```python
from build123d import *

# Parameters (mm, degrees)
SKETCH3_R                       = 4.7625
OXIDIZER_INLET_HOLE_DEPTH       = 102.060803604
FLANGE_HOLES_D                  = 5.1054
DOWEL_HOLES_D                   = 4.7625
DOWEL_HOLES_DEPTH               = 6.35
DOWEL_HOLES_TIP                 = 1.430799349
SKETCH12_R                      = 38.1
IMPINGING_PLATE_FLAT_CUT_DEPTH  = 3.81
SKETCH14_R                      = 38.1
SKETCH15_R                      = 38.1
SKETCH16_R                      = 28.575
SKETCH17_R                      = 4.7625
SKETCH21_R                      = 28.575
CUT_EXTRUDE1_DEPTH              = 9.525
INTERNAL_FILLET_R               = 3.175
EXTENDED_8_BC_COUNT             = 8
CHAMFER_FOR_IMPINGING_EDGE_SIZE = 0.127


with BuildPart() as part:
    # Sketch2 → Main Structure (revolve)
    with BuildSketch(Plane.XY, mode=Mode.PRIVATE) as main_structure_sk:
        Polygon((0, 0), (0, 63.5), (9.525, 63.5), (9.525, 45.72), (19.05, 45.72), (31.75, 13.081), (41.355, 13.081), (41.355, 6.2484), (46.355, 6.2484), (46.355, 0), align=None)
    revolve(main_structure_sk.sketch.rotate(Axis((0, 0, 0), (1, 0, 0)), 90), axis=Axis((0, 0, 0), (1, 0, 0)))

    # Sketch3 → Oxidizer Inlet Hole (cut, through all)
    with BuildSketch(Plane(origin=(46.355, 0, 0), x_dir=(0, 0, -1), z_dir=(1, 0, 0))):
        Circle(SKETCH3_R)
    extrude(amount=-OXIDIZER_INLET_HOLE_DEPTH, mode=Mode.SUBTRACT)

    # Flange Holes (through all)
    with Locations(Plane.ZY):
        with Locations((0, -58.42), (-29.21, -50.593204089), (-50.593204089, -29.21), (-58.42, 0), (-50.593204089, 29.21), (-29.21, 50.593204089), (0, 58.42), (29.21, 50.593204089), (50.593204089, 29.21), (58.42, 0), (50.593204089, -29.21), (29.21, -50.593204089)):
            Hole(FLANGE_HOLES_D / 2)

    # Dowel Holes
    with Locations(Plane.ZY):
        with Locations((56.429386772, -15.120208615), (-56.429386772, 15.120208615)):
            Hole(DOWEL_HOLES_D / 2, depth=DOWEL_HOLES_DEPTH)
            with Locations((0, 0, -(DOWEL_HOLES_DEPTH + DOWEL_HOLES_TIP / 2))):  # 118° drill point
                Cone(0, DOWEL_HOLES_D / 2, DOWEL_HOLES_TIP, mode=Mode.SUBTRACT)

    # Sketch12 → Impinging Plate Flat Cut (cut)
    with BuildSketch(Plane.ZY):
        Circle(SKETCH12_R)
    extrude(amount=-IMPINGING_PLATE_FLAT_CUT_DEPTH, mode=Mode.SUBTRACT)

    # Sketch14 → Impinging Plate Taper Cut section 0
    with BuildSketch(Plane.ZY.offset(-3.81)):
        Circle(SKETCH14_R)
    # Sketch15 → Impinging Plate Taper Cut section 1
    with BuildSketch(Plane.ZY.offset(-6.35)):
        Circle(SKETCH15_R)
    loft(mode=Mode.SUBTRACT)

    # Sketch16 → Internal Flow Path Loft Cut section 0
    with BuildSketch(Plane.ZY.offset(-15.875)):
        Circle(SKETCH16_R)
    # Sketch17 → Internal Flow Path Loft Cut section 1
    with BuildSketch(Plane.ZY.offset(-31.115)):
        Circle(SKETCH17_R)
    loft(mode=Mode.SUBTRACT)

    # Sketch21 → Cut-Extrude1 (cut)
    with BuildSketch(Plane.ZY.offset(-6.35)):
        Circle(SKETCH21_R)
    extrude(amount=-CUT_EXTRUDE1_DEPTH, mode=Mode.SUBTRACT)

    # Internal Fillet
    internal_fillet_edges = [part.edges().sort_by_distance(p)[0] for p in [
        (31.115, 4.7625, 0),
    ]]
    fillet(internal_fillet_edges, radius=INTERNAL_FILLET_R)

    # Sketch20 → 4-40 Tapped Holes (revolve, cut)
    with BuildSketch(Plane(origin=(6.35, 0, 33.3375), x_dir=(0, 0, 1), z_dir=(0, 1, 0))):
        Polygon((0, 0), (0, 13.887152758), (1.1303, 13.208), (1.1303, 0), align=None)
    f_4_40_tapped_holes = revolve(axis=Axis((0, 0, 33.3375), (1, 0, 0)), mode=Mode.SUBTRACT)

    # Extended 8 BC: 4-40 Tapped Holes ×8 about axis
    extended_8_bc_axis = Axis((0, 0, 0), (1, 0, 0))
    for i in range(1, EXTENDED_8_BC_COUNT):
        add(f_4_40_tapped_holes.rotate(extended_8_bc_axis, i * 360 / EXTENDED_8_BC_COUNT), mode=Mode.SUBTRACT)

    # Chamfer for Impinging Edge
    chamfer_for_impinging_edge_edges = [part.edges().sort_by_distance(p)[0] for p in [
        (6.35, 0, -38.1),
    ]]
    chamfer(chamfer_for_impinging_edge_edges, length=CHAMFER_FOR_IMPINGING_EDGE_SIZE)


solid = part.part
```
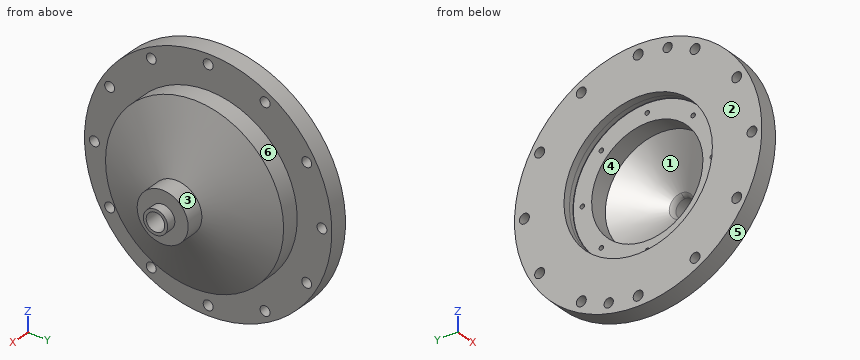
The model under review builds one solid part; all positions refer to its coordinate system, in mm. Face numbers are marked on the shaded views. A direction names the side the tool comes from. Give positions to 0.01 mm unless a question says otherwise; leave off trailing zeros. Write each loop counter-clockwise with the first axis right and the second up, starting at its lowest first coordinate (ties: lowest second). Pieces come first, ordered by that corner, then holes. Notation, with made-up numbers: M -39,45.5 L -3,45.5 A24 cw -3,60.5 Z; hole C -35.5,-24.75 d2. An arc over 180 degrees is marked long. Write each question's results on one line, items separated by ' | '. Start each with the question number.
1. For probe 1 along Y at (x, z) = (5, 0); probe 2 along Y at (x, z) = (34, 0.5); probe 3 along Y at (x, z) = (5.5, 31), list the stretches that pass through material, from the lowest coordinate up. Write a range as [from, to].
2. Mouldability with a two-part tool opening along Y and no side actions: class the marked faces 1, 2 and 3 as released by +Y, released by -Y, zero draft, split by the parting line, or undercut.
3. We need section A-A (y = -58.42). Write out the cut boundary in (x, z) (3 decimals).
4. Insertion check: pin 1 Ø4.5 at (y, z) = (-50.59, -29.21) entering from +X; pin 2 Ø1.4 at (y, z) = (23.57, -23.57) entering from +X; pin 3 Ø4 at (y, z) = (15.12, -56.43) entering from +X (3 decimals); pin 4 Ø3 at (y, z) = (-1, 46.5) entering from +X. Each pin has a flat end and moves straight along its axis. Give the tip position at first contact, or say it passes through.
5. For the marked faces 4, 5 and 6, list the 3-axis set-ups (+Z, -Z, +X, -X, +Y, -Y) from which the entire face can be reached by the end or side of a thin tool; tool diameter is ignored.
Results found:
1) probe 1: y = [-63.5, -60.97], [-55.87, -38.1], [38.1, 55.87], [60.97, 63.5] | probe 2: y = [-13.07, -4.74], [4.74, 13.07] | probe 3: y = [-55.42, -52.41], [-48.77, -22.15], [22.15, 48.77], [52.41, 55.42]
2) face 1: undercut | face 2: zero draft | face 3: split by the parting line
3) outline: M 0,-24.887 L 9.525,-24.887 L 9.525,-2.553 L 0,-2.553 Z; M 0,2.553 L 9.525,2.553 L 9.525,24.887 L 0,24.887 Z
4) pin 1: passes through | pin 2: stops at x = 24.14 | pin 3: stops at x = 9.525 | pin 4: stops at x = 19.33
5) face 4: -X | face 5: +X, -X | face 6: +X
